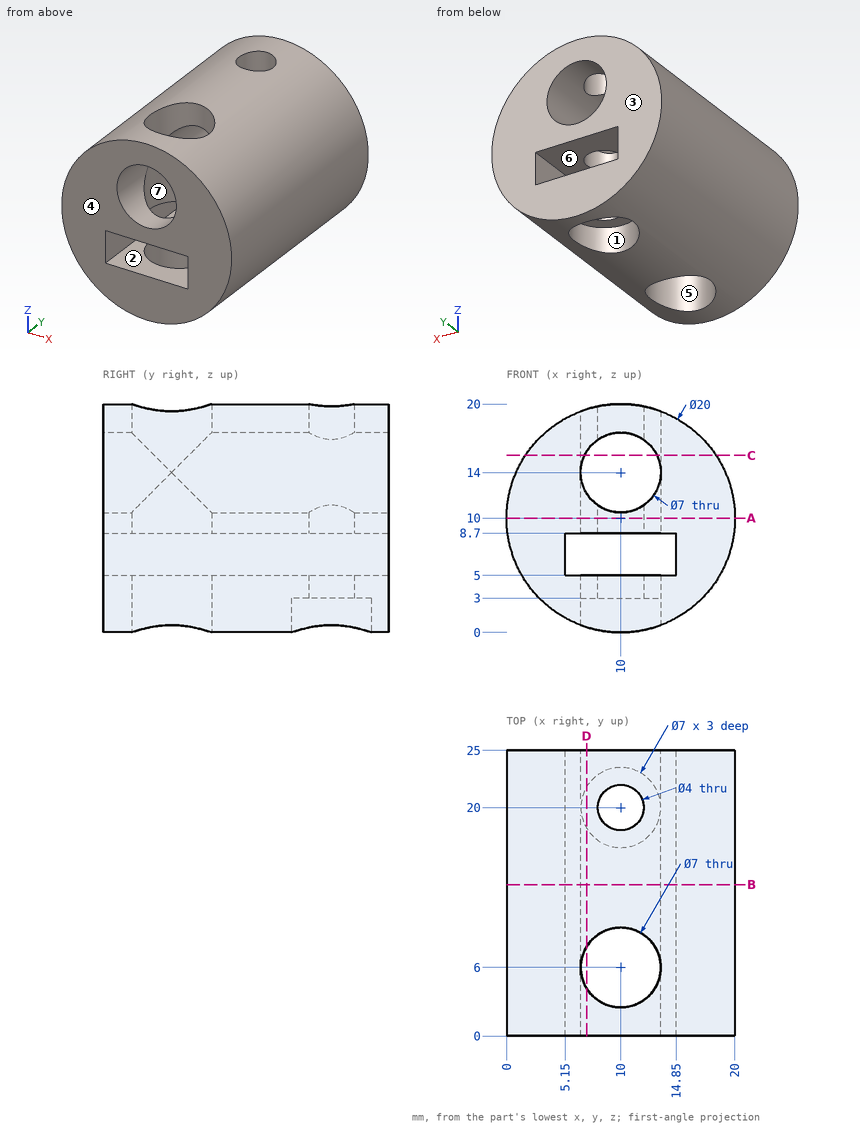
Print and shaded views of the part. All mm, measured from the part's lowest x, y and z. A direction names the side the tool comes from. Coordinates: 2 decimals unless noted, no trailing zeros. Loops run counter-clockwise (first coordinate to the right, second up) from the corner with the lowest first, then second, coordinate; pieces in that order, holes last. Notation, with made-up numbers: M -11.75,5.25 L 4.25,5.25 A33 cw 4.25,42.25 Z; hole C 44.25,68.25 d2. An arc over 180 degrees is marked long. Use a Markdown table: item, result. Add a question column.
Q1. Cut at C-C (z = 15.5). Write the cut outline in (x, y), and give its area (3 significant figures).
Q2. Cut at D-D (x = 7). Write the cut outline in (y, z).
Q3. Cut at B-B (y = 13.25). Write the cut outline in (x, z).
Q4. Which spindle directions (+Z, -Z, +X, -X, +Y, -Y) get a long thin tool onto all of the face, cutting with end or side? Do the marked faces 1, 2 and 3. Say none if no direction does.
Q5. Mould opens along Y. For the marked faces 4, 5, 6 and 7 say: +Y half, -Y half, draft (parallel to the pull), parting line (faces both ways), or undercut.
Q6. Cut at A-A (z = 10). Write the cut outline in (x, y), and give its area (3 significant figures).
Q7. Probe L1, parallel to Y at x = 10, z = 2.55; L2, parallel to Z at x = 8.25, y = 14.75; L3, parallel to X at y = 20.25, z = 6.75. List the from-to ranges inside material, lowest first.
Q8. Pin check, flat tips, straight feed: P1, Ø4, axis at x = 7.5, z = 8.5, coming from the -Y side; P2, Ø3, axis at y = 11, z = 7.5, coming from the -X side; P3, Ø1.1, axis at y = 12, z = 7, coming from the +X side; P4, Ø4.5, axis at x = 10, y = 20, coming from the -Z side. Stop position of each tip, or through.
Worked out:
| question | item | result |
|---|---|---|
| 1 | outline | M 1.65,0 L 6.84,0 L 6.84,4.5 A3.5 cw 6.84,7.5 L 6.84,25 L 1.65,25 Z; M 13.16,0 L 18.35,0 L 18.35,25 L 13.16,25 L 13.16,7.5 A3.5 cw 13.16,4.5 Z |
| 1 | area | 258 mm2 |
| 2 | outline | M 0,0.46 L 4.2,0.46 L 4.2,5 L 0,5 Z; M 0,8.7 L 4.2,8.7 L 4.2,12.2 L 0,12.2 Z; M 0,15.8 L 4.2,15.8 L 4.2,19.54 L 0,19.54 Z; M 7.8,0.46 L 18.2,0.46 L 18.2,3 L 21.8,3 L 21.8,0.46 L 25,0.46 L 25,5 L 7.8,5 Z; M 7.8,8.7 L 25,8.7 L 25,12.2 L 7.8,12.2 Z; M 7.8,15.8 L 25,15.8 L 25,19.54 L 7.8,19.54 Z |
| 3 | outline | C 10,10 d20; hole M 5.15,5 L 14.85,5 L 14.85,8.7 L 5.15,8.7 Z; hole C 10,14 d7 |
| 4 | face 1 | -Z |
| 4 | face 2 | +Y, -Y |
| 4 | face 3 | +Z, -Z, +X, -X, +Y |
| 5 | face 4 | -Y half |
| 5 | face 5 | undercut |
| 5 | face 6 | draft |
| 5 | face 7 | undercut |
| 6 | outline | M 0,0 L 20,0 L 20,25 L 0,25 Z; hole C 10,6 d7; hole C 10,20 d4 |
| 6 | area | 449 mm2 |
| 7 | L1 | y = 0 to 2.5, 9.5 to 16.5, 23.5 to 25 |
| 7 | L2 | z = 0.15 to 5, 8.7 to 10.97, 17.03 to 19.85 |
| 7 | L3 | x = 0.54 to 5.15, 14.85 to 19.46 |
| 8 | P1 | stops at y = 0 |
| 8 | P2 | stops at x = 0.05 |
| 8 | P3 | stops at x = 19.7 |
| 8 | P4 | stops at z = 3 |
